from build123d import *

# Parameters (mm, degrees)
SKETCH_1_R          = 1.4
EXTRUDE_1_DEPTH     = 2
SKETCH_2_R          = 2.5
EXTRUDE_2_DEPTH     = 18
CUT_EXTRUDE_START   = -3
SKETCH_3_R          = 1.4
CUT_EXTRUDE_1_DEPTH = 3


with BuildPart() as part:
    # 草图1 → 凸台-拉伸1 (new body)
    with BuildSketch(Plane(origin=(0, 0, 0), x_dir=(1, 0, 0), z_dir=(0, 1, 0))):
        with Locations(Location((0, 0, 0), (0, 0, 270))):
            Circle(SKETCH_1_R)
    extrude(amount=EXTRUDE_1_DEPTH)

    # 草图2 → 凸台-拉伸2 (add)
    with BuildSketch(Plane(origin=(0, 2, 0), x_dir=(1, 0, 0), z_dir=(0, 1, 0))):
        with Locations(Location((0, 0, 0), (0, 0, 270))):
            Circle(SKETCH_2_R)
    extrude(amount=EXTRUDE_2_DEPTH)

    # 草图3 → 切除-拉伸1 (cut)
    with BuildSketch(Plane(origin=(0, 20, 0), x_dir=(1, 0, 0), z_dir=(0, 1, 0)).offset(CUT_EXTRUDE_START)):
        with Locations(Location((0, 0, 0), (0, 0, 270))):
            Circle(SKETCH_3_R)
    extrude(amount=CUT_EXTRUDE_1_DEPTH, mode=Mode.SUBTRACT)


solid = part.part
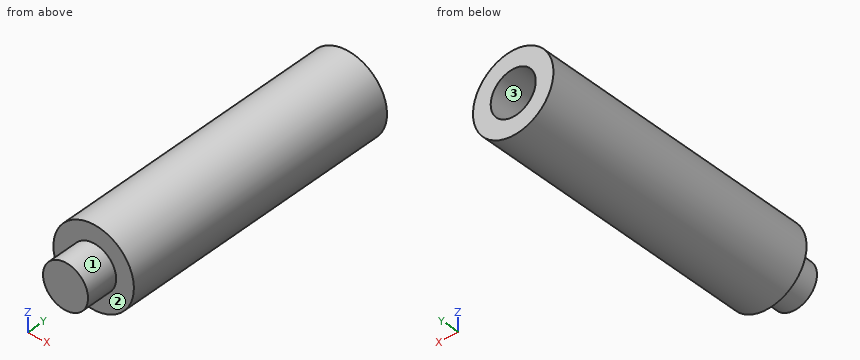
Design review of the part built by this model. Coordinates are the model's own, in mm. Face numbers are marked on the shaded views. Round coordinates to 2 decimals unless told otherwise and drop trailing zeros. Write each loop counter-clockwise with the first axis right and the second up, starting at its lowest first coordinate (ties: lowest second). Pieces come first, ordered by that corner, then holes. Notation, with made-up numbers: (-11.5, 9) -> (17.5, 9) arc R17 ccw to (17.5, 41) -> close; hole circle Ø5 at (-32.5, 14). An arc over 180 degrees is marked (long way). One line per item, written item: value. Start each with the question number.
Q1. Add section B-B (x = -0.35). Give the boundary of the cut face in (y, z), then the cut area to 3 significant figures.
Q2. To check wall thickness, follow probe 1 along X at (y, z) = (18, 0); probe 2 along Y at (x, z) = (1.6, -0.05); probe 3 along Y at (x, z) = (0.8, -0.8). State the ranges of each line that lie inside material, in increasing order.
Q3. Insertion check: P1, Ø2, axis at x = 0.5, z = 0, coming from the +Y side; P2, Ø1, axis at x = -0.5, z = 0, coming from the +Y side. Each pin has a flat end and moves straight along its axis. Give the tip position at first contact, or say it passes through.
Q4. Add section D-D (x = 1.8). Give the boundary of the cut face in (y, z), then the cut area to 3 significant figures.
Q5. The part is to be moulded in two halves that separate along Z. For the marked faces 1, 2 and 3, say which applies: pulls with the +Z half, pulls with the -Z half, needs draft (parallel to the pull), parting line crosses it, or undercut.
Q6. Add section C-C (y = 14.25). Give the boundary of the cut face in (x, z), then the cut area to 3 significant figures.
Q7. Add section A-A (z = 0). Give the boundary of the cut face in (x, y), then the cut area to 3 significant figures.
Response:
1. outline: (0, -1.36) -> (2, -1.36) -> (2, -2.48) -> (20, -2.48) -> (20, -1.36) -> (17, -1.36) -> (17, 1.36) -> (20, 1.36) -> (20, 2.48) -> (2, 2.48) -> (2, 1.36) -> (0, 1.36) -> close
1. area: 86.4 mm^2
2. probe 1: x = -2.5 to -1.4, 1.4 to 2.5
2. probe 2: y = 2 to 20
2. probe 3: y = 0 to 17
3. P1: stops at y = 20
3. P2: stops at y = 17
4. outline: (2, -1.73) -> (20, -1.73) -> (20, 1.73) -> (2, 1.73) -> close
4. area: 62.5 mm^2
5. face 1: parting line crosses it
5. face 2: needs draft
5. face 3: undercut
6. outline: circle Ø5 at (0, 0)
6. area: 19.6 mm^2
7. outline: (-2.5, 2) -> (-1.4, 2) -> (-1.4, 0) -> (1.4, 0) -> (1.4, 2) -> (2.5, 2) -> (2.5, 20) -> (1.4, 20) -> (1.4, 17) -> (-1.4, 17) -> (-1.4, 20) -> (-2.5, 20) -> close
7. area: 87.2 mm^2
